Could you check a few things on this model? Use its own coordinates, in mm. Round coordinates to 2 decimals unless told otherwise and drop trailing zeros. Write each loop counter-clockwise with the first axis right and the second up, starting at its lowest first coordinate (ties: lowest second). Pieces come first, ordered by that corner, then holes. Notation, with made-up numbers: (53.5, -7) -> (107.5, -7) arc R35 cw to (107.5, 32) -> close; hole circle Ø9 at (-17, 46.25). An arc over 180 degrees is marked (long way). One line per question, with ' | ' between items. Start each with the question number.
1. Imagine slicing it at A-A, the plane x = 12.7. List the corners of the cut face in (y, z) for me, and give its area (3 significant figures).
2. Thinking about a two-plate mould opening in X: for faces 1 (the cylindrical face through (-1.468, 6.439, -1.915)), 2 (the flat face through (-1, 6, -25.4)), 3 (the cylindrical face through (13.14, 6.261, -19.224)), 4 (the flat face through (-63.5, 6, 0)), which applies, released by +X, released by -X, zero draft, split by the parting line, or undercut?
3. If I drill on line 1 along Z through (x, y) = (-12.7, 5.75); line 2 along X through (y, z) = (6, -16); line 3 along Z through (x, y) = (-13, 8.5), over which ranges is the centre line in solid material (lowest first)? Write a range as [from, to].
4. Imagine slicing it at B-B, the plane y = 2. List the corners of the cut face in (x, z) for me (3 decimals).
from build123d import *

# Parameters (mm, degrees)
SKETCH1_W                 = 127
SKETCH1_H                 = 50.8
BOSS_EXTRUDE1_DEPTH       = 12.7
SKETCH2_R                 = 2.413
CUT_EXTRUDE1_DEPTH        = 70.560764803
F_1_4_CLEARANCE_HOLE1_D   = 6.7564
TAP_DRILL_FOR_8_32_TAP1_D = 3.4544


with BuildPart() as part:
    # Sketch1 → Boss-Extrude1 (new body)
    with BuildSketch(Plane(origin=(0, 0, 0), x_dir=(1, 0, 0), z_dir=(0, 1, 0))):
        Rectangle(SKETCH1_W, SKETCH1_H)
    extrude(amount=BOSS_EXTRUDE1_DEPTH)

    # Sketch2 → Cut-Extrude1 (cut, through all)
    with BuildSketch(Plane(origin=(0, 12.7, 0), x_dir=(1, 0, 0), z_dir=(0, 1, 0))):
        with Locations(Location((0, 0, 0), (0, 0, 270))):
            Circle(SKETCH2_R)
    extrude(amount=-CUT_EXTRUDE1_DEPTH, mode=Mode.SUBTRACT)

    # 1/4 Clearance Hole1 (through all)
    with Locations(Plane(origin=(0, 12.7, 0), x_dir=(1, 0, 0), z_dir=(0, 1, 0))):
        with Locations((-12.7, 15.875), (12.7, 15.875), (-12.7, -15.875), (12.7, -15.875)):
            Hole(F_1_4_CLEARANCE_HOLE1_D / 2)

    # Tap Drill for #8-32 Tap1 (through all)
    with Locations(Plane(origin=(0, 12.7, 0), x_dir=(1, 0, 0), z_dir=(0, 1, 0))):
        with Locations((12.7, 0), (-12.7, 0)):
            Hole(TAP_DRILL_FOR_8_32_TAP1_D / 2)


solid = part.part
Geometry results:
1) outline: (0, -25.4) -> (12.7, -25.4) -> (12.7, -19.25) -> (0, -19.25) -> close; (0, -12.5) -> (12.7, -12.5) -> (12.7, -1.73) -> (0, -1.73) -> close; (0, 1.73) -> (12.7, 1.73) -> (12.7, 12.5) -> (0, 12.5) -> close; (0, 19.25) -> (12.7, 19.25) -> (12.7, 25.4) -> (0, 25.4) -> close | area: 430 mm2
2) face 1: undercut | face 2: zero draft | face 3: undercut | face 4: released by -X
3) line 1: z = [-25.4, -19.25], [-12.5, -1.73], [1.73, 12.5], [19.25, 25.4] | line 2: x = [-63.5, -16.08], [-9.32, 9.32], [16.08, 63.5] | line 3: z = [-25.4, -19.24], [-12.51, -1.7], [1.7, 12.51], [19.24, 25.4]
4) outline: (-63.5, -25.4) -> (63.5, -25.4) -> (63.5, 25.4) -> (-63.5, 25.4) -> close; hole circle Ø6.756 at (-12.7, -15.875); hole circle Ø6.756 at (-12.7, 15.875); hole circle Ø3.454 at (-12.7, 0); hole circle Ø4.826 at (0, 0); hole circle Ø6.756 at (12.7, -15.875); hole circle Ø6.756 at (12.7, 15.875); hole circle Ø3.454 at (12.7, 0)
